Build history of the part. All positions in model axes, mm. A direction names the side the tool comes from. Round coordinates to 2 decimals unless told otherwise and drop trailing zeros. Loops run counter-clockwise (first coordinate to the right, second up) from the corner with the lowest first, then second, coordinate; pieces in that order, holes last. Notation, with made-up numbers: M 4,8.25 L 35,8.25 A27 ccw 35,26.25 Z; hole C 61,-9 d9. An arc over 180 degrees is marked long. One line per item, written item: value.
```python
from build123d import *

# Parameters (mm, degrees)
SKETCH1_W           = 40
SKETCH1_H           = 30
BOSS_EXTRUDE1_DEPTH = 8
SKETCH2_R           = 4.75
CUT_EXTRUDE1_DEPTH  = 7
SKETCH3_R           = 3.15
CUT_EXTRUDE2_DEPTH  = 5
SKETCH4_W           = 2.5
SKETCH4_H           = 2
CUT_EXTRUDE3_DEPTH  = 15


with BuildPart() as part:
    # Sketch1 → Boss-Extrude1 (new body)
    with BuildSketch(Plane(origin=(0, 0, 0), x_dir=(1, 0, 0), z_dir=(0, 1, 0))):
        with Locations((-20, 15)):
            Rectangle(SKETCH1_W, SKETCH1_H)
    extrude(amount=BOSS_EXTRUDE1_DEPTH)

    # Sketch2 → Cut-Extrude1 (cut)
    with BuildSketch(Plane(origin=(0, 8, 0), x_dir=(1, 0, 0), z_dir=(0, 1, 0))):
        with Locations(Location((-33, 24.5, 0), (0, 0, 270))):
            Circle(SKETCH2_R)
        with Locations(Location((-33, 5.5, 0), (0, 0, 90))):
            Circle(SKETCH2_R)
        with Locations(Location((-7, 5.5, 0), (0, 0, 270))):
            Circle(SKETCH2_R)
        with Locations(Location((-7, 24.5, 0), (0, 0, 90))):
            Circle(SKETCH2_R)
    extrude(amount=-CUT_EXTRUDE1_DEPTH, mode=Mode.SUBTRACT)

    # Sketch3 → Cut-Extrude2 (cut)
    with BuildSketch(Plane.XZ):
        with Locations(Location((-20, -15, 0), (0, 0, 270))):
            Circle(SKETCH3_R)
    extrude(amount=-CUT_EXTRUDE2_DEPTH, mode=Mode.SUBTRACT)

    # Sketch4 → Cut-Extrude3 (cut)
    with BuildSketch(Plane.XZ):
        with Locations((-12.75, -1)):
            Rectangle(SKETCH4_W, SKETCH4_H)
        with Locations((-27.25, -1)):
            Rectangle(SKETCH4_W, SKETCH4_H)
        with Locations((-12.75, -29)):
            Rectangle(SKETCH4_W, SKETCH4_H)
        with Locations((-27.25, -29)):
            Rectangle(SKETCH4_W, SKETCH4_H)
    extrude(amount=-CUT_EXTRUDE3_DEPTH, mode=Mode.SUBTRACT)


solid = part.part
```
Item 1: Slice it at B-B, the plane z = -5.5. Give the cut face in (x, y), and give its area (3 significant figures).
Check values:
outline: M -40,0 L 0,0 L 0,8 L -2.25,8 L -2.25,1 L -11.75,1 L -11.75,8 L -28.25,8 L -28.25,1 L -37.75,1 L -37.75,8 L -40,8 Z
area: 187 mm2
Item 2: Slice it at C-C, the plane x = -7. Give the cut face in (y, z), and give its area (3 significant figures).
Check values:
outline: M 0,-30 L 8,-30 L 8,-29.25 L 1,-29.25 L 1,-19.75 L 8,-19.75 L 8,-10.25 L 1,-10.25 L 1,-0.75 L 8,-0.75 L 8,0 L 0,0 Z
area: 107 mm2
Item 3: Slice it at A-A, the plane y = 2.5. Give the cut face in (x, z).
Check values:
outline: M -40,-30 L -28.5,-30 L -28.5,-28 L -26,-28 L -26,-30 L -14,-30 L -14,-28 L -11.5,-28 L -11.5,-30 L 0,-30 L 0,0 L -11.5,0 L -11.5,-2 L -14,-2 L -14,0 L -26,0 L -26,-2 L -28.5,-2 L -28.5,0 L -40,0 Z; hole C -33,-24.5 d9.5; hole C -33,-5.5 d9.5; hole C -20,-15 d6.3; hole C -7,-24.5 d9.5; hole C -7,-5.5 d9.5
Item 4: Drop flat-ended pins along their axis: P1, Ø0.6, axis at y = 3.5, z = -0.5, coming from the +X side; P2, Ø3, axis at x = -8, z = -6, coming from the +Y side. Give the stop position or say it passes through.
Check values:
P1: stops at x = 0
P2: stops at y = 1
Item 5: Slice it at D-D, the plane z = -15. Give the cut face in (x, y), and give its area (4 significant figures).
Check values:
outline: M -40,0 L -23.15,0 L -23.15,5 L -16.85,5 L -16.85,0 L 0,0 L 0,8 L -40,8 Z
area: 288.5 mm2
Item 6: Pull direction X, two halves, no side cores. Call faces 4 (the face through (0, 4, -15)), 5 (the face through (-26, 4, -29)), 6 (the face through (-20, 4, -30)): pulls with the +X half, pulls with the -X half, needs draft (parallel to the pull), parting line crosses it, or undercut.
Check values:
face 4: pulls with the +X half
face 5: undercut
face 6: needs draft
Item 7: Which spindle directions (+Z, -Z, +X, -X, +Y, -Y) get a long thin tool onto all of the face, cutting with end or side? Do faces 1 (the face through (-7, 1, -24)), 2 (the face through (-28.5, 4, -29)), 3 (the face through (-26, 4, -1)). Say none if no direction does.
Check values:
face 1: +Y
face 2: -Z, +Y, -Y
face 3: +Z, +Y, -Y
Item 8: Wall check: line 1 along X through (y, z) = (3, -5.5); line 2 along X through (y, z) = (1.9, -15); line 3 along Z through (x, y) = (-35, 4.5). Give the ranges that are in metal, low to high.
Check values:
line 1: x = -40 to -37.75, -28.25 to -11.75, -2.25 to 0
line 2: x = -40 to -23.15, -16.85 to 0
line 3: z = -30 to -28.81, -20.19 to -9.81, -1.19 to 0
